```python
from build123d import *

# Parameters (mm, degrees)
SKETCH1_W           = 228.6
SKETCH1_H           = 152.4
BOSS_EXTRUDE1_DEPTH = 80
SHELL1_T            = -2
SKETCH2_W           = 236.6
SKETCH2_H           = 160.4
SKETCH2_W_2         = 224.6
SKETCH2_H_2         = 148.4
BOSS_EXTRUDE2_DEPTH = 10
CHAMFER1_SIZE       = 2


with BuildPart() as part:
    # Sketch1 → Boss-Extrude1 (new body)
    with BuildSketch(Plane(origin=(0, 0, 0), x_dir=(1, 0, 0), z_dir=(0, 1, 0))):
        with Locations((114.3, 76.2)):
            Rectangle(SKETCH1_W, SKETCH1_H)
    extrude(amount=BOSS_EXTRUDE1_DEPTH)

    # Shell1
    shell1_openings = [part.faces().sort_by_distance(p)[0] for p in [
        (114.3, 80, -76.2),
    ]]
    offset(amount=SHELL1_T, openings=shell1_openings, kind=Kind.INTERSECTION)

    # Sketch2 → Boss-Extrude2 (add)
    with BuildSketch(Plane(origin=(0, 80, 0), x_dir=(1, 0, 0), z_dir=(0, 1, 0))):
        with Locations((114.3, 76.2)):
            Rectangle(SKETCH2_W, SKETCH2_H)
        with Locations((114.3, 76.2)):
            Rectangle(SKETCH2_W_2, SKETCH2_H_2, mode=Mode.SUBTRACT)
    extrude(amount=-BOSS_EXTRUDE2_DEPTH)

    # Chamfer1
    chamfer1_edges = [part.edges().sort_by_distance(p)[0] for p in [
        (114.3, 70, -152.4),
        (0, 70, -76.2),
        (114.3, 70, 0),
        (228.6, 70, -76.2),
        (114.3, 70, 4),
        (-4, 70, -76.2),
        (114.3, 70, -156.4),
        (232.6, 70, -76.2),
    ]]
    chamfer(chamfer1_edges, length=CHAMFER1_SIZE - 0.0001)  # a hair under: the kernel refuses the full size


solid = part.part
```
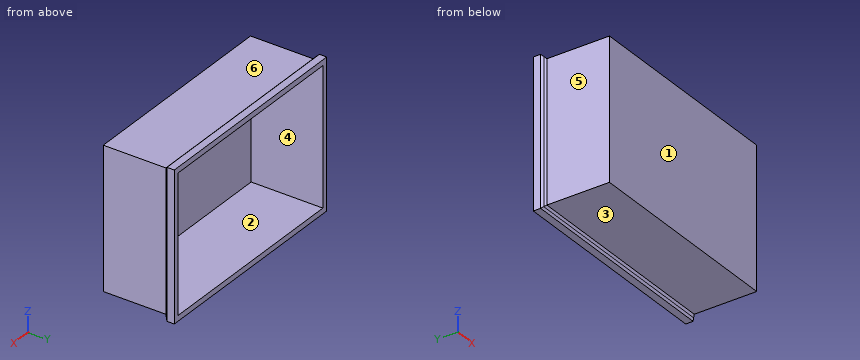
Design review of the part built by this model. Coordinates are the model's own, in mm. Face numbers are marked on the shaded views. A direction names the side the tool comes from. Round coordinates to 2 decimals unless told otherwise and drop trailing zeros. Write each loop counter-clockwise with the first axis right and the second up, starting at its lowest first coordinate (ties: lowest second). Pieces come first, ordered by that corner, then holes.
Item 1: The part is to be moulded in two halves that separate along Z. For the marked faces 1, 2 and 3, say which applies: +Z half, -Z half, draft (parallel to the pull), parting line (faces both ways), or undercut.
Item 2: Clearance check with flat-ended pins moving along their axes: pin 1 Ø3 at (x, z) = (58, -113) entering from +Y; pin 2 Ø4 at (x, y) = (32, 59.5) entering from +Z; pin 3 Ø10 at (x, z) = (170, -19) entering from -Y; pin 4 Ø10 at (y, z) = (66.5, -88) entering from -X. State where each tip first meets the part, or that it passes through.
Item 3: For probe 1 along Z at (x, y) = (63, 26); probe 2 along X at (y, z) = (10, -101.5); probe 3 along Z at (x, y) = (68.5, 74), list the stretches that pass through material, from the lowest coordinate up.
Item 4: We need section A-A on y = 32. Write out the cut boundary in (x, z).
Item 5: For the marked faces 4, 5 and 6, list the 3-axis set-ups (+Z, -Z, +X, -X, +Y, -Y) from which the entire face can be reached by the end or side of a thin tool; tool diameter is ignored.
Returned:
1. face 1: draft
1. face 2: undercut
1. face 3: -Z half
2. pin 1: stops at y = 2
2. pin 2: stops at z = 0
2. pin 3: stops at y = 0
2. pin 4: stops at x = -3.5
3. probe 1: z = -152.4 to -150.4, -2 to 0
3. probe 2: x = 0 to 2, 226.6 to 228.6
3. probe 3: z = -156.4 to -150.4, -2 to 4
4. outline: (0, -152.4) - (228.6, -152.4) - (228.6, 0) - (0, 0) - close; hole (2, -150.4) - (226.6, -150.4) - (226.6, -2) - (2, -2) - close
5. face 4: +Y
5. face 5: +Z, -Z, -X, -Y
5. face 6: +Z, +X, -X, -Y
